Read the model definition and answer for the solid it produces. Units are mm, in the model's axes. A direction names the side the tool comes from. Coordinates: 2 decimals unless noted, no trailing zeros. Loops run counter-clockwise (first coordinate to the right, second up) from the corner with the lowest first, then second, coordinate; pieces in that order, holes last. Notation, with made-up numbers: (-8.5, -14.75) -> (28.5, -14.75) arc R32 ccw to (28.5, 22.25) -> close; hole circle Ø4 at (74.5, 0.25). An arc over 180 degrees is marked (long way). One line per question, with ' | ' between items. Start each with the question number.
```python
from build123d import *

# Parameters (mm, degrees)
ESQUISSE1_W             = 20
ESQUISSE1_H             = 40
BOSS_EXTRU_1_DEPTH      = 5
CONG_1_R                = 10
CONG_2_R                = 10
ESQUISSE2_R             = 2.5
ENL_V_MAT_EXTRU_1_DEPTH = 10


with BuildPart() as part:
    # Esquisse1 → Boss.-Extru.1 (new body)
    with BuildSketch(Plane.XY):
        with BuildLine():
            Line((-8.855638783, 10), (24.569838787, 10))
            ThreePointArc((24.569838787, 10), (30.866124306, -45.477583457), (7.330413731, -96.108362687))
            ThreePointArc((7.330413731, -96.108362687), (1.361276776, -97.354484204), (-1.373289466, -91.904203266))
            ThreePointArc((-1.373289466, -91.904203266), (-0.740706025, -65.321594201), (-8.855638783, -40))
            Line((-8.855638783, -40), (-8.855638783, 10))
        make_face()
        with Locations((10, -20)):
            Rectangle(ESQUISSE1_W, ESQUISSE1_H, mode=Mode.SUBTRACT)
    extrude(amount=BOSS_EXTRU_1_DEPTH)

    # Congé1
    cong_1_edges = [part.edges().sort_by_distance(p)[0] for p in [
        (24.569838787, 10, 2.5),
    ]]
    fillet(cong_1_edges, radius=CONG_1_R)

    # Congé2
    cong_2_edges = [part.edges().sort_by_distance(p)[0] for p in [
        (-8.855638783, -40, 2.5),
        (-8.855638783, 10, 2.5),
    ]]
    fillet(cong_2_edges, radius=CONG_2_R)

    # Esquisse2 → Enlèv. mat.-Extru.1 (cut)
    with BuildSketch(Plane.XY.offset(5)):
        with Locations((4.5, 5)):
            Circle(ESQUISSE2_R)
        with Locations((15.5, 5)):
            Circle(ESQUISSE2_R)
        with Locations((4.5, -45)):
            Circle(ESQUISSE2_R)
        with Locations((15.5, -45)):
            Circle(ESQUISSE2_R)
    extrude(amount=-ENL_V_MAT_EXTRU_1_DEPTH, mode=Mode.SUBTRACT)


solid = part.part
```
(1) Section C-C on y = -32.5 is taken. Write down the section's boundary in (x, z), plus the area to 3 significant figures.
(2) A tool of negligible diameter and unlimited length cuts with its end or side. For faces 4 (the cylindrical face through (-0.544, -66.778, 2.465)), 5 (the flat face through (10, 0, 2)), from which of +Z, -Z, +X, -X, +Y, -Y can it reach the whole face along a straight path? Write none if from no direction.
(3) Section A-A on x = 4.5 is taken. Write down the section's boundary in (y, z), plus the area to 3 significant figures.
(4) Each of these flat-tipped pins is pushed along its axis until it touches: pin 1 Ø6.5 at (x, y) = (15.5, -45) entering from +Z; pin 2 Ø3 at (y, z) = (-30, 1) entering from +X; pin 3 Ø1.5 at (x, z) = (10.5, 2) entering from -Y; pin 4 Ø2 at (x, z) = (18.5, 4.5) entering from -Y. Where does it stop, or does it pass through?
(5) Section D-D on z = 2.8 is taken. Write down the section's boundary in (x, y).
(6) Determine the mould class of faces 1 (the cylindrical face through (1.44, -97.39, 2.46)), 2 (the flat face through (0, -20, 2)), 3 (the flat face through (9, 10, 2)) for opening direction X: +X half, -X half, draft (parallel to the pull), parting line (faces both ways), or undercut.
(7) Section B-B on y = 5 is taken. Write down the section's boundary in (x, z), plus the area to 3 significant figures.
(8) Find the intervals of material crossed by probe 1 along Y at (x, z) = (4.5, 3.3); probe 2 along Y at (x, z) = (14.5, 1.8); probe 3 along X at (y, z) = (-46, 2.7), in increasing order. Write a range as from..to.
Working result:
1) outline: (-8.86, 0) -> (0, 0) -> (0, 5) -> (-8.86, 5) -> close; (20, 0) -> (32.14, 0) -> (32.14, 5) -> (20, 5) -> close | area: 105 mm2
2) face 4: +Z, -Z, -X | face 5: +Z, -Z
3) outline: (-97.76, 0) -> (-47.5, 0) -> (-47.5, 5) -> (-97.76, 5) -> close; (-42.5, 0) -> (-40, 0) -> (-40, 5) -> (-42.5, 5) -> close; (0, 0) -> (2.5, 0) -> (2.5, 5) -> (0, 5) -> close; (7.5, 0) -> (10, 0) -> (10, 5) -> (7.5, 5) -> close | area: 289 mm2
4) pin 1: stops at z = 5 | pin 2: stops at x = 32.2 | pin 3: stops at y = -93.18 | pin 4: stops at y = -82.01
5) outline: (-8.86, -37.64) arc R10 ccw to (-7.86, -41.99) arc R80 cw to (-1.37, -91.9) arc R5 ccw to (7.33, -96.11) arc R103.15 ccw to (27.1, 3.11) arc R10 ccw to (17.59, 10) -> (1.14, 10) arc R10 ccw to (-8.86, 0) -> close; hole (0, -40) -> (20, -40) -> (20, 0) -> (0, 0) -> close; hole circle Ø5 at (4.5, -45); hole circle Ø5 at (4.5, 5); hole circle Ø5 at (15.5, -45); hole circle Ø5 at (15.5, 5)
6) face 1: parting line | face 2: undercut | face 3: draft
7) outline: (-7.52, 0) -> (2, 0) -> (2, 5) -> (-7.52, 5) -> close; (7, 0) -> (13, 0) -> (13, 5) -> (7, 5) -> close; (18, 0) -> (26.25, 0) -> (26.25, 5) -> (18, 5) -> close | area: 119 mm2
8) probe 1: y = -97.76..-47.5, -42.5..-40, 0..2.5, 7.5..10 | probe 2: y = -86.71..-47.29, -42.71..-40, 0..2.71, 7.29..10 | probe 3: x = -6.06..2.21, 6.79..13.21, 17.79..30.78
